```python
from build123d import *

# Parameters (mm, degrees)
F1_DEPTH  = 203.2
F2_DEPTH  = 6.35
F3_R      = 19.05
F6_DEPTH  = 101.6
F4_R      = 19.05
F7_DEPTH  = 101.6
F5_R      = 19.05
F8_DEPTH  = 101.6
F10_DEPTH = 25.4


with BuildPart() as f1:
    # F0 (on Top) → F1 (new body)
    with BuildSketch(Plane.XY):
        Polygon((25.6632194655, 44.45), (-25.6632194655, 44.45), (-51.326438931, 0), (-25.6632194655, -44.45), (25.6632194655, -44.45), (51.326438931, 0), align=None)
        Polygon((43.9940905122, 0), (21.9970452561, -38.1), (-21.9970452561, -38.1), (-43.9940905122, 0), (-21.9970452561, 38.1), (21.9970452561, 38.1), align=None, mode=Mode.SUBTRACT)
    extrude(amount=F1_DEPTH)

    # F0 (on Top) → F2 (join)
    with BuildSketch(Plane.XY):
        Polygon((-21.9970452561, -38.1), (21.9970452561, -38.1), (43.9940905122, 0), (21.9970452561, 38.1), (-21.9970452561, 38.1), (-43.9940905122, 0), align=None)
    extrude(amount=F2_DEPTH)

    # F3 (on face) → F6 (cut)
    with BuildSketch(Plane.XZ.offset(44.45)):
        with BuildLine():
            ThreePointArc((0, 194.056), (-13.4703841816, 161.5356158184), (19.05, 175.006))
            ThreePointArc((19.05, 175.006), (13.4703841816, 188.4763841816), (0, 194.056))
        make_face()
        with Locations((0, 131.11192)):
            Circle(F3_R)
        with Locations((0, 87.21784)):
            Circle(F3_R)
        with Locations((0, 43.32376)):
            Circle(F3_R)
    extrude(amount=-F6_DEPTH, mode=Mode.SUBTRACT)

    # F4 (on face) → F7 (cut)
    with BuildSketch(Plane(origin=(38.4948291982, -22.225, 0), x_dir=(0.5, 0.8660254038, 0), z_dir=(0.8660254038, -0.5, 0))):
        with BuildLine():
            ThreePointArc((0, 194.056), (-13.4703841816, 161.5356158184), (19.05, 175.006))
            ThreePointArc((19.05, 175.006), (13.4703841816, 188.4763841816), (0, 194.056))
        make_face()
        with Locations((0, 130.78592)):
            Circle(F4_R)
        with Locations((0, 86.56584)):
            Circle(F4_R)
        with Locations((0, 42.34576)):
            Circle(F4_R)
    extrude(amount=-F7_DEPTH, mode=Mode.SUBTRACT)

    # F5 (on face) → F8 (cut)
    with BuildSketch(Plane(origin=(-38.4948291982, -22.225, 0), x_dir=(0.5, -0.8660254038, 0), z_dir=(-0.8660254038, -0.5, 0))):
        with BuildLine():
            ThreePointArc((0, 194.056), (-13.4703841816, 161.5356158184), (19.05, 175.006))
            ThreePointArc((19.05, 175.006), (13.4703841816, 188.4763841816), (0, 194.056))
        make_face()
        with Locations((0, 130.41386)):
            Circle(F5_R)
        with Locations((0, 85.82172)):
            Circle(F5_R)
        with Locations((0, 41.22958)):
            Circle(F5_R)
    extrude(amount=-F8_DEPTH, mode=Mode.SUBTRACT)

    # F9 (on face) → F10 (cut)
    with BuildSketch(Plane(origin=(0, 0, 0), x_dir=(1, 0, 0), z_dir=(0, 0, -1))):
        Polygon((-14.0039394503, -24.255534634), (14.0039394503, -24.255534634), (28.0078789005, 0), (14.0039394503, 24.255534634), (-14.0039394503, 24.255534634), (-28.0078789005, 0), align=None)
    extrude(amount=-F10_DEPTH, mode=Mode.SUBTRACT)


solid = f1.part
```
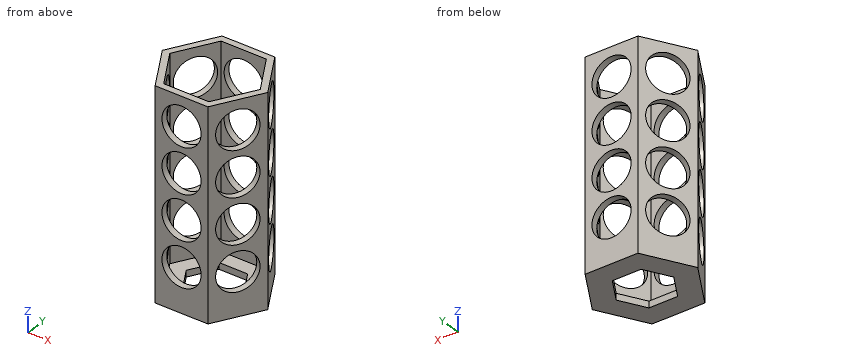
Can you work these out from the model? Positions are in its coordinate system, mm. Coordinates: 2 decimals unless noted, no trailing zeros. Return JSON: item names as keys, results as strings.
Q1. Please list where these lines run through material, in increasing order: L1, parallel to Z at x = 0, y = -42.5; L2, parallel to Y at x = -20.5, z = 171; L3, parallel to Z at x = 26, y = 6. Write a range as from..to.
Computed values:
{"L1": "z = 0..24.27, 62.37..68.17, 106.27..112.06, 150.16..155.96, 194.06..203.2", "L2": "y = -44.45..-38.1, 38.1..44.45", "L3": "z = 0..6.35"}
Q2. If we section it at A-A (x = 0): Count the separate pieces of the cut face and the enclosed holes in it, then the cut area to 3 significant figures.
Computed values:
{"separate pieces": "10", "enclosed holes": "0", "area": "821 mm2"}
Q3. I'm going to push flat-ended pins straight in: pin 1 Ø4 at (y, z) = (-24, 148.5) entering from -X; pin 2 Ø5 at (x, z) = (30.5, 113) entering from -Y; pin 3 Ø3 at (x, y) = (23, 16) entering from +Z. Where does each tip first touch, or does it pass through?
Computed values:
{"pin 1": "stops at x = -38.48", "pin 2": "stops at y = -40.4", "pin 3": "stops at z = 6.35"}
